Read the model definition and answer for the solid it produces. Units are mm, in the model's axes. A direction names the side the tool comes from. Coordinates: 2 decimals unless noted, no trailing zeros. Write each loop counter-clockwise with the first axis right and the second up, starting at its lowest first coordinate (ties: lowest second). Pieces come first, ordered by that corner, then holes. Notation, with made-up numbers: (-6, -18.75) - (1, -18.75) arc R20 cw to (1, 5.25) - close; hole circle Ø8 at (36.25, 60.25). An arc over 180 degrees is marked (long way). Use a Markdown table: item, result.
from build123d import *

# Parameters (mm, degrees)
SKETCH1_W           = 151.3
SKETCH1_H           = 127
BOSS_EXTRUDE1_DEPTH = 18
SKETCH3_W           = 18
SKETCH3_H           = 127
CUT_EXTRUDE2_DEPTH  = 6.35
SKETCH2_W           = 151.3
SKETCH2_H           = 18
CUT_EXTRUDE3_DEPTH  = 6.35


with BuildPart() as part:
    # Sketch1 → Boss-Extrude1 (new body)
    with BuildSketch(Plane(origin=(0, 0, 0), x_dir=(1, 0, 0), z_dir=(0, 1, 0))):
        Rectangle(SKETCH1_W, SKETCH1_H)
    extrude(amount=BOSS_EXTRUDE1_DEPTH)

    # Sketch3 → Cut-Extrude2 (cut)
    with BuildSketch(Plane(origin=(0, 18, 0), x_dir=(1, 0, 0), z_dir=(0, 1, 0))):
        with Locations((66.65, 0)):
            Rectangle(SKETCH3_W, SKETCH3_H)
        with Locations((-66.65, 0)):
            Rectangle(SKETCH3_W, SKETCH3_H)
    extrude(amount=-CUT_EXTRUDE2_DEPTH, mode=Mode.SUBTRACT)

    # Sketch2 → Cut-Extrude3 (cut)
    with BuildSketch(Plane(origin=(0, 18, 0), x_dir=(1, 0, 0), z_dir=(0, 1, 0))):
        with Locations((0, -54.5)):
            Rectangle(SKETCH2_W, SKETCH2_H)
        with Locations((0, 54.5)):
            Rectangle(SKETCH2_W, SKETCH2_H)
    extrude(amount=-CUT_EXTRUDE3_DEPTH, mode=Mode.SUBTRACT)


solid = part.part
(1) Each of these flat-tipped pins is pushed along its axis until it touches: P1, Ø7, axis at x = 0, y = 16, coming from the -Z side; P2, Ø1.9, axis at y = 16.5, z = -9, coming from the -X side; P3, Ø1.9, axis at x = -10.5, y = 14, coming from the +Z side; P4, Ø4, axis at x = -58, z = 44.5, coming from the +Y side. Where does it stop, or does it pass through?
Report:
| item | result |
|---|---|
| P1 | stops at z = -45.5 |
| P2 | stops at x = -57.65 |
| P3 | stops at z = 45.5 |
| P4 | stops at y = 18 |
(2) A cutting plane is placed at C-C, the plane y = 14.75. Write down the section's boundary in (x, z).
Report:
| item | result |
|---|---|
| outline | (-57.65, -45.5) - (57.65, -45.5) - (57.65, 45.5) - (-57.65, 45.5) - close |
(3) A cutting plane is placed at B-B, the plane z = 21.5. Write down the section's boundary in (x, y).
Report:
| item | result |
|---|---|
| outline | (-75.65, 0) - (75.65, 0) - (75.65, 11.65) - (57.65, 11.65) - (57.65, 18) - (-57.65, 18) - (-57.65, 11.65) - (-75.65, 11.65) - close |
(4) Straight lines are drawn through the part: L1, parallel to Z at x = -20.5, y = 14.75; L2, parallel to Y at x = -18, z = -55; L3, parallel to X at y = 13.5, z = 44. For each, find the intervals that lie inside material, in ascending order.
Report:
| item | result |
|---|---|
| L1 | z = -45.5 to 45.5 |
| L2 | y = 0 to 11.65 |
| L3 | x = -57.65 to 57.65 |
(5) For faces 1 (the flat face through (-57.65, 15, 1)), 2 (the flat face through (-1, 15, 45.5)), 3 (the flat face through (57.65, 15, 1)), 4 (the flat face through (-1, 15, -45.5)), determine the directions among +Z, -Z, +X, -X, +Y, -Y from which every point of the face is accessible in a straight line to the end or side of a thin tool.
Report:
| item | result |
|---|---|
| face 1 | +Z, -Z, -X, +Y |
| face 2 | +Z, +X, -X, +Y |
| face 3 | +Z, -Z, +X, +Y |
| face 4 | -Z, +X, -X, +Y |
(6) A cutting plane is placed at A-A, the plane x = -54. Write down the section's boundary in (y, z).
Report:
| item | result |
|---|---|
| outline | (0, -63.5) - (11.65, -63.5) - (11.65, -45.5) - (18, -45.5) - (18, 45.5) - (11.65, 45.5) - (11.65, 63.5) - (0, 63.5) - close |
(7) A cutting plane is placed at D-D, the plane z = -48. Write down the section's boundary in (x, y), and give its area (3 significant figures).
Report:
| item | result |
|---|---|
| outline | (-75.65, 0) - (75.65, 0) - (75.65, 11.65) - (-75.65, 11.65) - close |
| area | 1,760 mm² |
